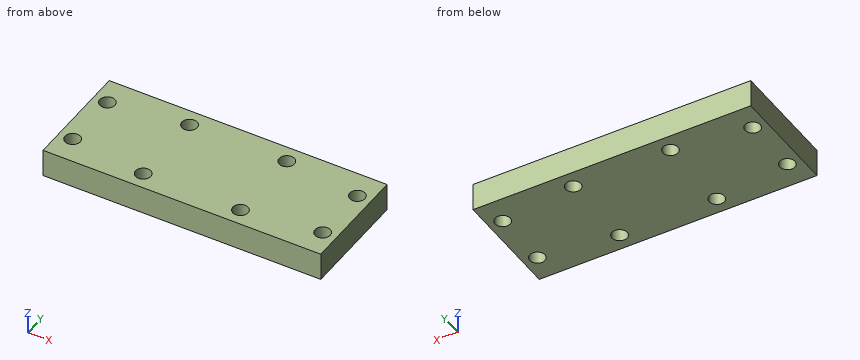
Autodesk Inventor part; units mm, degrees
ref_plane "YZ Plane" through (0, 0, 0) normal (1, 0, 0) x (0, 1, 0)
ref_plane "XZ Plane" through (0, 0, 0) normal (0, 1, 0) x (-1, 0, 0)
ref_plane "XY Plane" through (0, 0, 0) normal (0, 0, 1) x (1, 0, 0)
sketch "Sketch1" plane through (0, 0, 0) normal (0, 0, 1) x (1, 0, 0)
  line L0 (-50, 20) -> (50, 20)
  line L1 (50, 20) -> (50, -20)
  line L2 (50, -20) -> (-50, -20)
  line L3 (-50, -20) -> (-50, 20)
  circle A0 centre (-45, 10.5) radius 2.75
  circle A1 centre (-45, -10.5) radius 2.75
  circle A2 centre (45, 10.5) radius 2.75
  circle A3 centre (45, -10.5) radius 2.75
  line L4 (-45, 10.5) -> (-45, -10.5) construction
  point P0 (0, 0)
  point P1 (-50, 0)
  point P2 (0, 20)
  point P3 (-45, 0)
  dimension "d0" = 40
  dimension "d1" = 100
  dimension "d2" = 5.5
  dimension "d3" = 5.5
  dimension "d4" = 5
  dimension "d7" = 5
  dimension "d10" = 90
  dimension "d29" = 21
sketch "Sketch2" plane through (0, 0, 0) normal (0, 0, 1) x (1, 0, 0)
  circle A0 centre (-17.5, 14) radius 2.75
  circle A1 centre (17.5, 14) radius 2.75
  line L0 (-17.5, 14) -> (17.5, 14) construction
  line L1 (0, 0) -> (0, 14) construction
  circle A2 centre (-17.5, -14) radius 2.75
  circle A3 centre (17.5, -14) radius 2.75
  dimension "d15" = 5.5
  dimension "d17" = 5.5
  dimension "d20" = 35
  dimension "d21" = 14
  dimension "d24" = 28
extrude "Extrusion1" add sketch "Sketch1" against normal blind 10
extrude "Extrusion2" cut sketch "Sketch2" against normal through all
properties part number "casterplate"
Design review of the part built by this model. Coordinates are the model's own, in mm. Round coordinates to 2 decimals unless told otherwise and drop trailing zeros. Order: outer loops, then holes, each group sorted by start corner. A loop starts at its lowest first (then second) coordinate and runs counter-clockwise, first axis right, second up. Notation, with made-up numbers: M -28.75,75.5 L -19.75,75.5 A23 ccw -19.75,88.5 Z; hole C -20.75,36 d8. An arc over 180 degrees is marked long. Put each result on its own line as item: value.
Q1. To check wall thickness, follow line 1 (Y direction, x = 45, z = -4.25); line 2 (Y direction, x = 19, z = -3.25); line 3 (X direction, y = 16, z = -3.75). State the ranges of each line that lie inside material, in increasing order.
Reported:
line 1: -20 to -13.25, -7.75 to 7.75, 13.25 to 20
line 2: -20 to -16.3, -11.7 to 11.7, 16.3 to 20
line 3: -50 to -19.39, -15.61 to 15.61, 19.39 to 50
Q2. Consider section A-A (z = -3.75). State how many separate pieces and enclosed holes the cut face has, and give its area (3 significant figures).
Reported:
separate pieces: 1
enclosed holes: 8
area: 3,810 mm²
Q3. Consider section B-B (x = -45). State the section outline as (y, z) points, and give its area (3 significant figures).
Reported:
outline: M -20,-10 L -13.25,-10 L -13.25,0 L -20,0 Z; M -7.75,-10 L 7.75,-10 L 7.75,0 L -7.75,0 Z; M 13.25,-10 L 20,-10 L 20,0 L 13.25,0 Z
area: 290 mm²
